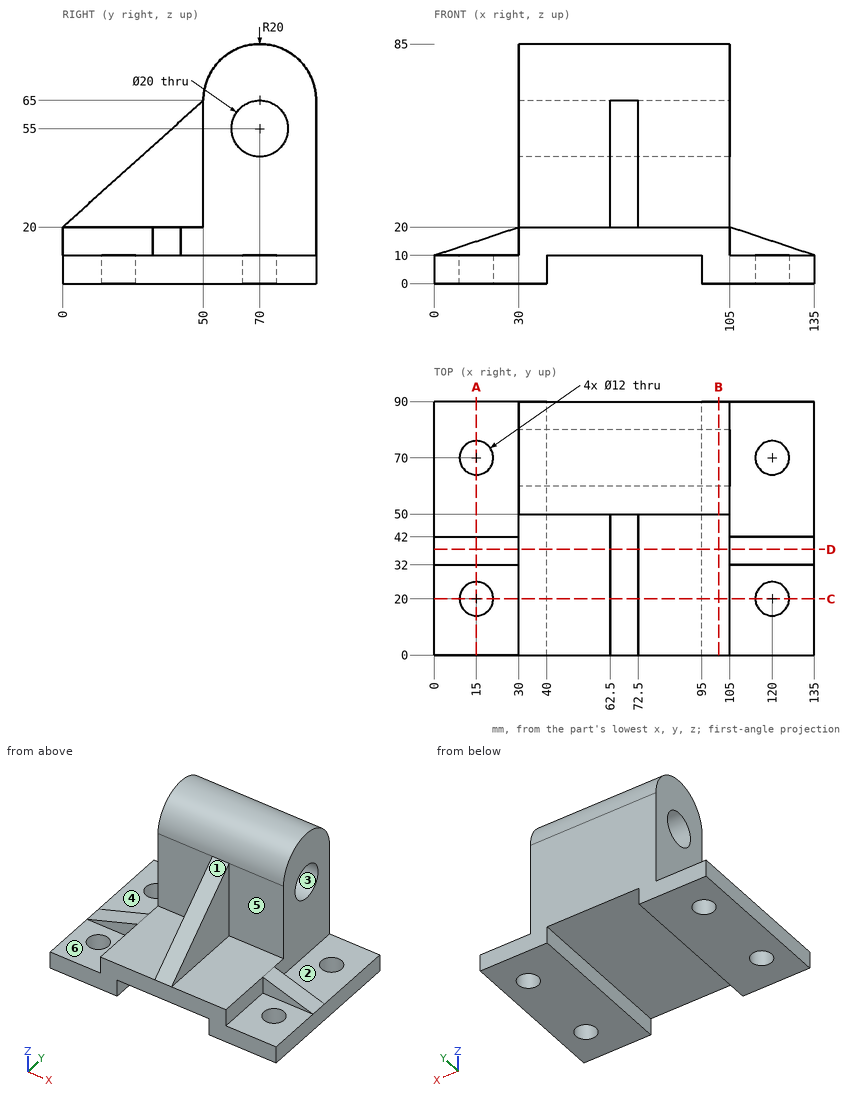
Answer from the drawing. Dimensions are ordinates in mm from the lowest x, y and z of the part. A direction names the side the tool comes from. Give positions to 0.01 mm unless a question says otherwise; leave off trailing zeros. Order: outer loops, then holes, each group sorted by start corner. A loop starts at its lowest first (then second) coordinate and runs counter-clockwise, first axis right, second up.
Item 1: The part is cut by section D-D, the plane y = 37.5. Give the vertices of the cut face in (x, z).
From the geometry:
outline: (0, 0) - (40, 0) - (40, 10) - (95, 10) - (95, 0) - (135, 0) - (135, 10) - (105, 20) - (72.5, 20) - (72.5, 53.75) - (62.5, 53.75) - (62.5, 20) - (30, 20) - (0, 10) - close
Item 2: Find the intervals of material crossed by probe 1 along Y at (x, z) = (15, 7.5); probe 2 along Y at (x, z) = (83, 54.5); probe 3 along Z at (x, y) = (54, 43.5), in increasing order.
From the geometry:
probe 1: y = 0 to 14, 26 to 64, 76 to 90
probe 2: y = 50 to 60.01, 79.99 to 90
probe 3: z = 10 to 20
Item 3: Given pin 1 Ø2 at (x, y) = (37, 33) entering from +Z; pin 2 Ø15 at (x, y) = (13, 11) entering from +Z; pin 3 Ø12 at (x, y) = (56.5, 36.5) entering from -Z; pin 4 Ø6 at (x, y) = (42.5, 17) entering from -Z, each flat-ended and moving along its own axis, determine where each tip first touches the part or whether it passes through.
From the geometry:
pin 1: stops at z = 20
pin 2: stops at z = 10
pin 3: stops at z = 10
pin 4: stops at z = 0
Item 4: The part is cut by section C-C, the plane y = 20. Give the vertices of the cut face in (x, z).
From the geometry:
outline: (0, 0) - (9, 0) - (9, 10) - (0, 10) - close; (21, 0) - (40, 0) - (40, 10) - (95, 10) - (95, 0) - (114, 0) - (114, 10) - (105, 10) - (105, 20) - (72.5, 20) - (72.5, 38) - (62.5, 38) - (62.5, 20) - (30, 20) - (30, 10) - (21, 10) - close; (126, 0) - (135, 0) - (135, 10) - (126, 10) - close
Item 5: The part is cut by section B-B, the plane x = 101. Give the vertices of the cut face in (y, z), and give its area (3 significant figures).
From the geometry:
outline: (0, 0) - (90, 0) - (90, 65) arc R20 ccw to (50, 65) - (50, 20) - (0, 20) - close; hole circle Ø20 at (70, 55)
area: 3,910 mm2
Item 6: The part is cut by section A-A, the plane x = 15. Give the vertices of the cut face in (y, z), and give its area (3 significant figures).
From the geometry:
outline: (0, 0) - (14, 0) - (14, 10) - (0, 10) - close; (26, 0) - (64, 0) - (64, 10) - (42, 10) - (42, 15) - (32, 15) - (32, 10) - (26, 10) - close; (76, 0) - (90, 0) - (90, 10) - (76, 10) - close
area: 710 mm2
Item 7: For a pull along Y with two mould halves and no side action, classify the marked faces 1, 2 and 3 as pulls with the +Y half, pulls with the -Y half, needs draft (parallel to the pull), parting line crosses it, or undercut.
From the geometry:
face 1: pulls with the -Y half
face 2: needs draft
face 3: undercut
Item 8: Which of the six approach directions +Z, -Z, +X, -X, +Y, -Y give full straight-line access (tool end or side, diameter ignored) to the marked faces 4, 5 and 6?
From the geometry:
face 4: +Z, -X, +Y
face 5: +Z, +X, -Y
face 6: +Z, -X, -Y
